The listing builds one solid part. Answer for the finished solid, in the listing's coordinates (mm). A direction names the side the tool comes from. Round coordinates to 2 decimals unless told otherwise and drop trailing zeros. Loops run counter-clockwise (first coordinate to the right, second up) from the corner with the lowest first, then second, coordinate; pieces in that order, holes last. Notation, with made-up numbers: M 53.5,48.25 L 60.5,48.25 A37 cw 60.5,84.25 Z; hole C 67,-30 d3. An arc over 180 degrees is marked long. Put each result on its own line as item: value. Start each with the question number.
(1) Determine the mould class of faces 6 (the face through (5, 1, 5)), 7 (the face through (-22.5, 3, 14)), 8 (the face through (14.4, 0.8, -23.5)) for opening direction Z: released by +Z, released by -Z, zero draft, split by the parting line, or undercut.
(2) Section D-D, the plane z = 8 is taken. Determine the outline of the cut face in (x, y).
(3) Section B-B, the plane y = 3.4 is taken. Determine the outline of the cut face in (x, z), then the cut area to 3 significant figures.
(4) Section A-A, the plane z = -20 is taken. Determine the outline of the cut face in (x, y).
(5) Straight lines are drawn through the part: line 1 (Z direction, x = 5, y = 1.7); line 2 (X direction, y = 1.8, z = 18.5); line 3 (X direction, y = 4.2, z = -16). For each, find the intervals that lie inside material, in ascending order.
(6) Section C-C, the plane x = 15.5 is taken. Determine the outline of the cut face in (y, z), then the cut area to 3 significant figures.
(7) Flat-ended cylindrical pins translate along their axes: P1, Ø13, axis at x = 3.5, z = -11.5, coming from the +Y side; P2, Ø5, axis at x = 8.5, z = 17.5, coming from the +Y side; P3, Ø1.2, axis at x = 4.5, y = 4, coming from the -Z side. Find the tip coordinate at first contact, or state that the pin passes through.
(8) Which of the six approach directions +Z, -Z, +X, -X, +Y, -Y give full straight-line access (tool end or side, diameter ignored) to faces 1 (the face through (-13.5, 3, 18)), 2 (the face through (0, 2, -18.5)), 3 (the face through (-4, 3, 4.5)), 4 (the face through (0, 0, 0)), 5 (the face through (22.5, 3, -6))?
Autodesk Inventor part; units mm, degrees
ref_plane "YZ Plane" through (0, 0, 0) normal (1, 0, 0) x (0, 1, 0)
ref_plane "XZ Plane" through (0, 0, 0) normal (0, 1, 0) x (-1, 0, 0)
ref_plane "XY Plane" through (0, 0, 0) normal (0, 0, 1) x (1, 0, 0)
sketch "Sketch1" plane through (0, 0, 0) normal (0, 1, 0) x (-1, 0, 0)
  point P0 (0, 0)
sketch "Sketch2" plane through (0, 0, 0) normal (0, 1, 0) x (-1, 0, 0)
  line L0 (23.5, 23.5) -> (-23.5, 23.5)
  line L1 (-23.5, 23.5) -> (-23.5, -23.5)
  line L2 (23.5, -23.5) -> (23.5, 23.5)
  line L3 (8.5, -18.5) -> (-8.5, -18.5)
  line L4 (-8.5, -23.5) -> (-8.5, -18.5)
  line L5 (8.5, -18.5) -> (8.5, -23.5)
  line L6 (-23.5, -23.5) -> (-8.5, -23.5)
  line L7 (8.5, -23.5) -> (23.5, -23.5)
  point P0 (0, 0)
  dimension "d4" = 47
  dimension "d5" = 47
  dimension "d7" = 23.5
  dimension "d41" = 15
  dimension "d42" = 15
extrude "Extrusion1" add sketch "Sketch2" along normal blind 5
sketch "Sketch3" plane through (0, 5, 0) normal (0, 1, 0) x (1, 0, 0)
  point P0 (0, 0)
sketch "Sketch4" plane through (0, 5, 0) normal (0, 1, 0) x (1, 0, 0)
  line L0 (22.5, -22.5) -> (22.5, 22.5)
  line L1 (-22.5, 22.5) -> (-22.5, -31.5)
  line L2 (22.5, 22.5) -> (13.5356, 22.5)
  line L3 (22.5, 11) -> (22.5, 22.5)
  line L4 (13.5, -4.5) -> (-22.5, -4.5)
  line L5 (-22.5, -4.5) -> (-22.5, -23.5)
  line L6 (-23.5, 23.5) -> (-23.5, -23.5)
  line L7 (-22.5, -23.5) -> (-13.5, -23.5)
  line L8 (-13.5, -23.5) -> (-13.5, -11.5)
  line L9 (-13.5, -11.5) -> (22.5, -11.5)
  line L10 (13.5, -4.5) -> (13.5, 23.5)
  line L11 (13.5, 23.5) -> (22.5, 23.5)
  line L12 (22.5, 23.5) -> (22.5, -11.5)
  line L13 (22.5, -22.5) -> (-12.5, -22.5)
  line L14 (-12.5, -22.5) -> (-12.5, -12.5)
  line L15 (-12.5, -12.5) -> (22.5, -12.5)
  line L16 (22.5, -12.5) -> (22.5, -22.5)
  line L17 (12.5, 22.5) -> (12.5, -3.5)
  line L18 (12.5, -3.5) -> (-22.5, -3.5)
  line L19 (-22.5, -3.5) -> (-22.5, 22.5)
  line L20 (-9.5, 22.5) -> (-9.5, 17.5)
  line L21 (-9.5, 17.5) -> (9.5, 17.5)
  line L22 (9.5, 17.5) -> (9.5, 22.5)
  line L23 (-8.5, 18.5) -> (-8.5, 23.5)
  line L24 (8.5, 23.5) -> (8.5, 18.5)
  line L25 (22.5, 22.5) -> (8.5, 22.5)
  line L26 (-8.5, 22.5) -> (-22.5, 22.5)
  line L27 (-22.5, 22.5) -> (-8.5, 22.5)
  line L28 (8.5, 22.5) -> (12.5, 22.5)
  line L29 (-5, -3.5) -> (-20.0496, -3.5)
  line L30 (-20.0496, -3.5) -> (-20.0496, 2.4851)
  line L31 (-20.0496, 2.4851) -> (-5, 2.4851)
  line L32 (-5, 2.4851) -> (-5, -3.5)
  line L33 (-23.5, -23.5) -> (23.5, -23.5)
  line L34 (23.5, 23.5) -> (8.5, 23.5)
  point P0 (0, 0)
  point P1 (22.5, 22.5)
  point P2 (22.5, -12.5)
  point P3 (-22.5, -3.5)
  point P4 (-9.5, 20)
  point P5 (8.5, 21)
  point P6 (12.5, 22.5)
  point P7 (13.5, 22.5)
  point P8 (9.5, 22.5)
  point P9 (22.5, 22.5)
  point P10 (10.5, 22.5)
  dimension "d10" = 45
  dimension "d13" = 22.5
  dimension "d33" = 9
  dimension "d36" = 1
  dimension "d38" = 1
  dimension "d39" = 1
  dimension "d43" = 5
  dimension "d44" = 1
  dimension "d45" = 1
  dimension "d50" = 1
  dimension "d51" = 11
  dimension "d52" = 18
  dimension "d53" = 1
  dimension "d54" = 1
extrude "Extrusion5" cut sketch "Sketch4" against normal blind 4 contours L13 L14 L15 L0 | L9 L8 L7 L1 L4 L10 L25 L2 L0 | L2 L25 L10 L11 L12 | L17 L18 L32 L31 L30 L1 L26 L20 L21 L22 L25 | L30 L31 L32 L18
sketch "PD placement" plane through (0, 1, 0) normal (0, 1, 0) x (1, 0, 0)
  line L0 (-4.5, -10.5) -> (0, -10.5)
  line L1 (0, -10.5) -> (0, -5)
  line L2 (0, -5) -> (-4.5, -5)
  line L3 (-4.5, -5) -> (-4.5, -10.5)
  line L4 (22.5, -22.5) -> (-12.5, -22.5)
  line L5 (22.5, 23.5) -> (22.5, -11.5)
  line L6 (-22.5, -23.5) -> (-22.5, -4.5)
  point P0 (0, 0)
  dimension "d55" = 4.5
  dimension "d56" = 5.5
  dimension "d57" = 12
  dimension "d59" = 18
properties part number "particle_sensor_case_top"
Recorded:
1. face 6: undercut
1. face 7: zero draft
1. face 8: released by -Z
2. outline: M -23.5,0 L 23.5,0 L 23.5,5 L 22.5,5 L 22.5,1 L -22.5,1 L -22.5,5 L -23.5,5 Z
3. outline: M -23.5,-23.5 L -8.5,-23.5 L -8.5,-18.5 L 8.5,-18.5 L 8.5,-23.5 L 13.5,-23.5 L 13.5,4.5 L -22.5,4.5 L -22.5,23.5 L -23.5,23.5 Z; M -13.5,11.5 L 22.5,11.5 L 22.5,-23.5 L 23.5,-23.5 L 23.5,23.5 L -13.5,23.5 Z; hole M -22.5,-22.5 L -9.5,-22.5 L -9.5,-17.5 L 9.5,-17.5 L 9.5,-22.5 L 12.5,-22.5 L 12.5,3.5 L -22.5,3.5 Z; hole M -12.5,12.5 L 22.5,12.5 L 22.5,22.5 L -12.5,22.5 Z
3. area: 284 mm²
4. outline: M -23.5,0 L -8.5,0 L -8.5,5 L -9.5,5 L -9.5,1 L -22.5,1 L -22.5,5 L -23.5,5 Z; M 8.5,0 L 23.5,0 L 23.5,5 L 22.5,5 L 22.5,1 L 13.5,1 L 13.5,5 L 12.5,5 L 12.5,1 L 9.5,1 L 9.5,5 L 8.5,5 Z
5. line 1: z = -18.5 to -17.5, 3.5 to 4.5, 11.5 to 12.5, 22.5 to 23.5
5. line 2: x = -23.5 to -22.5, -13.5 to -12.5, 22.5 to 23.5
5. line 3: x = -23.5 to -22.5, 12.5 to 13.5, 22.5 to 23.5
6. outline: M 0,-23.5 L 1,-23.5 L 1,11.5 L 5,11.5 L 5,12.5 L 1,12.5 L 1,22.5 L 5,22.5 L 5,23.5 L 0,23.5 Z
6. area: 55.0 mm²
7. P1: stops at y = 5
7. P2: stops at y = 1
7. P3: stops at z = -18.5
8. face 1: +Z, +Y
8. face 2: -Z, +Y, -Y
8. face 3: +Y
8. face 4: +Z, -Z, +X, -X, -Y
8. face 5: -Z, +Y
